CAD build for the part. Positions are in the model's coordinates, mm. Face numbers are marked on the shaded views. A direction names the side the tool comes from. Give positions to 0.01 mm unless a question says otherwise; leave off trailing zeros. Write each loop counter-clockwise with the first axis right and the second up, starting at its lowest first coordinate (ties: lowest second). Pieces come first, ordered by that corner, then holes. Notation, with made-up numbers: (-36, 10) - (-3, 10) arc R25 ccw to (-3, 43) - close; hole circle Ø3 at (86, -17.75). An arc over 180 degrees is marked (long way). Answer as a JSON object with one key per item and string values.
from build123d import *

# Parameters (mm, degrees)
F5_W            = 1
F5_H            = 9
F6_DEPTH        = 15
F6_COPIES_COUNT = 8
F7_W            = 1.7910775183
F7_H            = 2
F8_DEPTH        = 17.2
F8_COPIES_COUNT = 8


# Not quite as in the source:
# - a fillet or chamfer that OpenCascade refuses, or shapes differently, is made with other operations: its cross-section is extruded or revolved along the edge and cut away or added
# - a pattern or mirror of a feature is missing from the dataset's text; its kind, count and spacing are read off the source's solid


with BuildPart() as f2:
    # F0 (on Front) → F2 (revolve)
    with BuildSketch(Plane.XZ):
        Polygon((-17.2, 0), (23.3, 0), (23.3, 5.5), (3.7, 5.5), (3.7, 9.5), (0, 9.5), (0, 8.6), (-17.2, 8.6), align=None)
    revolve(axis=Axis((3.6722049117, 0, 0), (1, 0, 0)))

    # F3 (on Front) → F4 (revolve, cut)
    with BuildSketch(Plane.XZ):
        Polygon((-17.2, 0), (23.3, 0), (23.3, 4.7), (20.6, 2), (0, 2), (0, 4), (-2.5, 4), (-2.5, 2), (-17.2, 2), align=None)
    revolve(axis=Axis((3.05, 0, 0), (1, 0, 0)), mode=Mode.SUBTRACT)

    # F5 (on face) → F6 (cut)
    with BuildSketch(Plane(origin=(-17.2, 0, 0), x_dir=(0, -1, 0), z_dir=(-1, 0, 0))):
        with Locations((0, 4.5)):
            Rectangle(F5_W, F5_H)
    f6 = extrude(amount=-F6_DEPTH, mode=Mode.SUBTRACT)

    # F6_copies: F6 ×8 about axis
    f6_copies_axis = Axis((0, 0, 0), (1, 0, 0))
    for i in range(1, F6_COPIES_COUNT):
        add(f6.rotate(f6_copies_axis, i * 360 / F6_COPIES_COUNT), mode=Mode.SUBTRACT)

    # F7 (on face) → F8 (cut, through all)
    with BuildSketch(Plane(origin=(-17.2, 0, 0), x_dir=(0, -1, 0), z_dir=(-1, 0, 0))):
        Polygon((4.7052910807, 9.359577542), (3.2910775183, 7.9453639796), (4.5575605772, 6.6788809207), (5.9717741396, 8.0930944831), align=None)
        with Locations((2.3955387592, 8.9453639796)):
            Rectangle(F7_W, F7_H)
    f8 = extrude(amount=-F8_DEPTH, mode=Mode.SUBTRACT)

    # F8_copies: F8 ×8 about axis
    f8_copies_axis = Axis((0, 0, 0), (1, 0, 0))
    for i in range(1, F8_COPIES_COUNT):
        add(f8.rotate(f8_copies_axis, i * 360 / F8_COPIES_COUNT), mode=Mode.SUBTRACT)

    # F9: fillet of radius 1 on 2 edges, made by hand

    # F9_s1 → F9_t2 (revolve, cut)
    with BuildSketch(Plane.XZ):
        with BuildLine():
            ThreePointArc((23.3, 4.7), (22.9526596349, 5.2745966692), (22.3202041029, 5.5))
            Line((22.3202041029, 5.5), (23.3, 5.5))
            Line((23.3, 5.5), (23.3, 4.7))
        make_face()
    revolve(axis=Axis((23.3, 0, 0), (1, 0, 0)), mode=Mode.SUBTRACT)

    # F9_s3 → F9_t4 (revolve, cut)
    with BuildSketch(Plane.XZ):
        with BuildLine():
            ThreePointArc((2.7, 9.5), (3.4071067812, 9.2071067812), (3.7, 8.5))
            Line((3.7, 8.5), (3.7, 9.5))
            Line((3.7, 9.5), (2.7, 9.5))
        make_face()
    revolve(axis=Axis((3.7, 0, 0), (1, 0, 0)), mode=Mode.SUBTRACT)


solid = f2.part
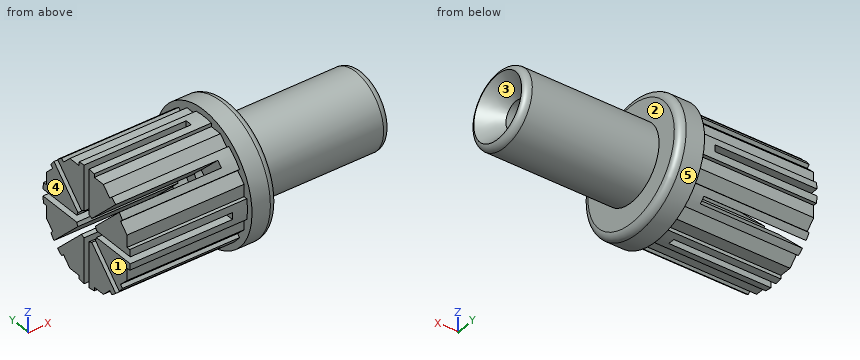
Item 1: Cut at D-D (x = -4.5). State how many separate pieces and enclosed holes the cut face has, and give its area (3 significant figures).
Entries:
{"separate pieces": "8", "enclosed holes": "0", "area": "158 mm2"}
Item 2: Cut at C-C (x = 11.5). Give the cut face in (y, z), and give its area (3 significant figures).
Entries:
{"outline": "circle Ø11 at (0, 0); hole circle Ø4 at (0, 0)", "area": "82.5 mm2"}
Item 3: Flat gauge pins, fed straight in: P1, Ø2, axis at x = 9.5, z = -4, coming from the -Y side; P2, Ø10, axis at x = -11, z = -1.5, coming from the -Y side; P3, Ø1, axis at y = 3, z = 1.5, coming from the +X side. Where does each tip first touch, or does it go through?
Entries:
{"P1": "y = -4.61", "P2": "y = -8.59", "P3": "x = 22.45"}
Item 4: Which spindle directions (+Z, -Z, +X, -X, +Y, -Y) get a long thin tool onto all of the face, cutting with end or side? Do the marked faces 1 and 2. Say none if no direction does.
Entries:
{"face 1": "+Z, -Z, -X, +Y, -Y", "face 2": "+X"}
Item 5: Mould opens along Y. For the marked faces 3, 4 and 5 say: +Y half, -Y half, draft (parallel to the pull), parting line (faces both ways), or undercut.
Entries:
{"face 3": "undercut", "face 4": "draft", "face 5": "parting line"}
Item 6: Cut at A-A (z = 0). Give the cut face in (x, y), and give its area (3 significant figures).
Entries:
{"outline": "(-2.2, -8.6) - (0, -8.6) - (0, -9.5) - (2.7, -9.5) arc R1 ccw to (3.7, -8.5) - (3.7, -5.5) - (22.32, -5.5) arc R1 ccw to (23.3, -4.7) - (20.6, -2) - (0, -2) - (0, -4) - (-2.2, -4) - close; (-2.2, 4) - (0, 4) - (0, 2) - (20.6, 2) - (23.3, 4.7) arc R1 ccw to (22.32, 5.5) - (3.7, 5.5) - (3.7, 8.5) arc R1 ccw to (2.7, 9.5) - (0, 9.5) - (0, 8.6) - (-2.2, 8.6) - close", "area": "205 mm2"}
Item 7: Probe line 1 (Z direction, x = 5, y = 0); line 2 (Y direction, x = -9, z = -8.25). List the from-to ranges inside material, lowest first. Write a range as from..to.
Entries:
{"line 1": "-5.5..-2, 2..5.5", "line 2": "-1.5..-0.5, 0.5..1.5"}
